from build123d import *

# Parameters (mm, degrees)
BOSS_EXTRUDE1_DEPTH = 42
SKETCH2_R           = 1.264493958
CUT_EXTRUDE1_DEPTH  = 50.879855653


with BuildPart() as part:
    # Sketch1 → Boss-Extrude1 (new body)
    with BuildSketch(Plane(origin=(0, 0, 0), x_dir=(0, 0, -1), z_dir=(1, 0, 0))):
        Polygon((0, 20), (0, 0), (20, 0), (20, 2), (2, 2), (2, 20), align=None)
    extrude(amount=-BOSS_EXTRUDE1_DEPTH)

    # Sketch2 → Cut-Extrude1 (cut, through all)
    with BuildSketch(Plane(origin=(0, 2, 0), x_dir=(1, 0, 0), z_dir=(0, 1, 0))):
        with Locations(Location((-21, 15.261871586, 0), (0, 0, 270))):
            Circle(SKETCH2_R)
        with Locations(Location((-16.738128414, 11, 0), (0, 0, 270))):
            Circle(SKETCH2_R)
        with Locations(Location((-21, 6.738128414, 0), (0, 0, 270))):
            Circle(SKETCH2_R)
        with Locations(Location((-25.261871586, 11, 0), (0, 0, 270))):
            Circle(SKETCH2_R)
    extrude(amount=-CUT_EXTRUDE1_DEPTH, mode=Mode.SUBTRACT)


solid = part.part
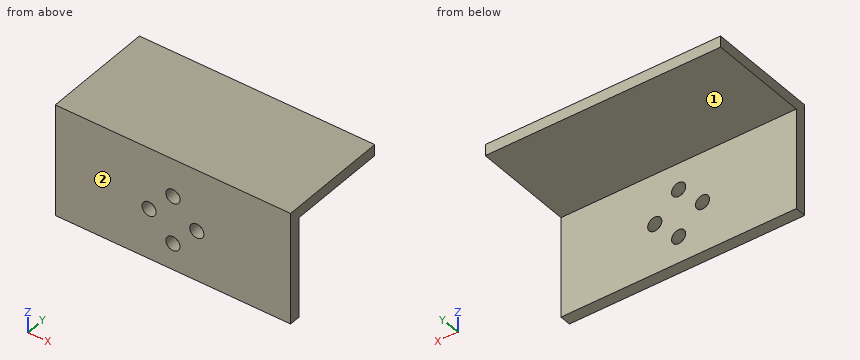
For this review, take the finished solid that the model builds, in its own axes (mm). Face numbers are marked on the shaded views. A direction names the side the tool comes from. Round coordinates to 2 decimals unless told otherwise and drop trailing zeros. Order: outer loops, then holes, each group sorted by start corner. A loop starts at its lowest first (then second) coordinate and runs counter-clockwise, first axis right, second up. Notation, with made-up numbers: (-10.5, 30) -> (35.5, 30) arc R36 ccw to (35.5, 67) -> close; hole circle Ø11 at (5.25, 30). An arc over 180 degrees is marked (long way). Write item = value, one per line. Start each with the question number.
1) Insertion check: pin 1 (4 mm diameter, centred on x = -12.5, z = -16.5, fed in from +Y); pin 2 (4 mm diameter, centred on x = -32, y = 4.5, fed in from -Z). Each pin has a flat end and moves straight along its axis. Give the tip position at first contact, or say it passes through.
2) To check wall thickness, follow line 1 (X direction, y = 0.4, z = -11); line 2 (Y direction, x = -27.5, z = -18.25); line 3 (Z direction, x = -22, y = 18). State the ranges of each line that lie inside material, in increasing order. Write a range as from..to.
3) Take a section at C-C on x = -11. State the section outline as (y, z) points.
4) Take a section at A-A on x = -21. State the section outline as (y, z) points, plus the area to 3 significant figures.
5) Take a section at B-B on z = -11. State the section outline as (x, y) points, plus the area to 3 significant figures.
6) Take a section at D-D on y = 4.25. State the section outline as (x, z) points.
7) Tool access review of the marked faces 1 and 2: name each direction out of +Z, -Z, +X, -X, +Y, -Y from which nothing blocks a thin tool from reaching the whole face with its end or side.
Verdict:
q1.pin_1 = 2
q1.pin_2 = -2
q2.line_1 = -42..-26.53, -24..-18, -15.47..0
q2.line_2 = 0..2
q2.line_3 = -2..0
q3.outline = (0, -20) -> (2, -20) -> (2, -2) -> (20, -2) -> (20, 0) -> (0, 0) -> close
q4.outline = (0, -20) -> (2, -20) -> (2, -16.53) -> (0, -16.53) -> close; (0, -14) -> (2, -14) -> (2, -8) -> (0, -8) -> close; (0, -5.47) -> (2, -5.47) -> (2, -2) -> (20, -2) -> (20, 0) -> (0, 0) -> close
q4.area = 65.9 mm2
q5.outline = (-42, 0) -> (-26.53, 0) -> (-26.53, 2) -> (-42, 2) -> close; (-24, 0) -> (-18, 0) -> (-18, 2) -> (-24, 2) -> close; (-15.47, 0) -> (0, 0) -> (0, 2) -> (-15.47, 2) -> close
q5.area = 73.9 mm2
q6.outline = (-42, -2) -> (0, -2) -> (0, 0) -> (-42, 0) -> close
q7.face_1 = -Z, +X, -X, +Y
q7.face_2 = +Z, -Z, +X, -X, -Y
